from build123d import *

# Parameters (mm, degrees)
SKETCH1_W           = 35
SKETCH1_H           = 20
BOSS_EXTRUDE4_DEPTH = 15
SHELL2_T            = -2
SKETCH8_R           = 1.5
BOSS_EXTRUDE7_DEPTH = 6.9
LPATTERN4_COUNT     = 3
LPATTERN4_PITCH     = 10.5
FILLET1_R           = 2
CUT_EXTRUDE2_START  = -5
SKETCH9_R           = 1.25
CUT_EXTRUDE2_DEPTH  = 34.469380611
SKETCH10_R          = 1.25
CUT_EXTRUDE3_DEPTH  = 28.311380776


with BuildPart() as part:
    # Sketch1 → Boss-Extrude4 (new body)
    with BuildSketch(Plane(origin=(0, 0, 0), x_dir=(1, 0, 0), z_dir=(0, 1, 0))):
        Rectangle(SKETCH1_W, SKETCH1_H)
    extrude(amount=BOSS_EXTRUDE4_DEPTH)

    # Shell2
    shell2_openings = [part.faces().sort_by_distance(p)[0] for p in [
        (0, 15, 0),
    ]]
    offset(amount=SHELL2_T, openings=shell2_openings, kind=Kind.INTERSECTION)

    # Sketch8 → Boss-Extrude7 (add)
    with BuildSketch(Plane(origin=(13.95, 0, 0), x_dir=(0, 0, -1), z_dir=(1, 0, 0))):
        with BuildLine():
            Line((13.926543174, 13.400522246), (10, 9))
            Line((10, 9), (10, 15))
            ThreePointArc((10, 15), (13.096526294, 16.982277643), (13.926543174, 13.400522246))
        make_face()
        with Locations((12.249990037, 14.993304126)):
            Circle(SKETCH8_R, mode=Mode.SUBTRACT)
    boss_extrude7 = extrude(amount=-BOSS_EXTRUDE7_DEPTH)

    # LPattern4: Boss-Extrude7 ×3
    with Locations(*[(-i * LPATTERN4_PITCH, 0, 0) for i in range(1, LPATTERN4_COUNT)]):
        add(boss_extrude7)

    # Fillet1
    fillet1_edges = [part.edges().sort_by_distance(p)[0] for p in [
        (17.5, 7.5, 10),
        (-17.5, 7.5, 10),
    ]]
    fillet(fillet1_edges, radius=FILLET1_R)

    # Sketch9 → Cut-Extrude2 (cut)
    with BuildSketch(Plane(origin=(0, 0, 0), x_dir=(1, 0, 0), z_dir=(0, 1, 0)).offset(CUT_EXTRUDE2_START)):
        with Locations(Location((-4.997517741, 4.250548665, 0), (0, 0, 90))):
            Circle(SKETCH9_R)
    cut_extrude2 = extrude(amount=CUT_EXTRUDE2_DEPTH, mode=Mode.SUBTRACT)

    # Sketch10 → Cut-Extrude3 (cut, through all)
    with BuildSketch(Plane(origin=(0, 2, 0), x_dir=(1, 0, 0), z_dir=(0, 1, 0))):
        with Locations(Location((-5.055245898, -0.559104904, 0), (0, 0, 270))):
            Circle(SKETCH10_R)
    cut_extrude3 = extrude(amount=-CUT_EXTRUDE3_DEPTH, mode=Mode.SUBTRACT)

    # Mirror1: Cut-Extrude2, Cut-Extrude3 across plane
    add(cut_extrude2.mirror(Plane(origin=(0, 0, 0), x_dir=(0, 0, 1), z_dir=(1, 0, 0))), mode=Mode.SUBTRACT)
    add(cut_extrude3.mirror(Plane(origin=(0, 0, 0), x_dir=(0, 0, 1), z_dir=(1, 0, 0))), mode=Mode.SUBTRACT)


solid = part.part
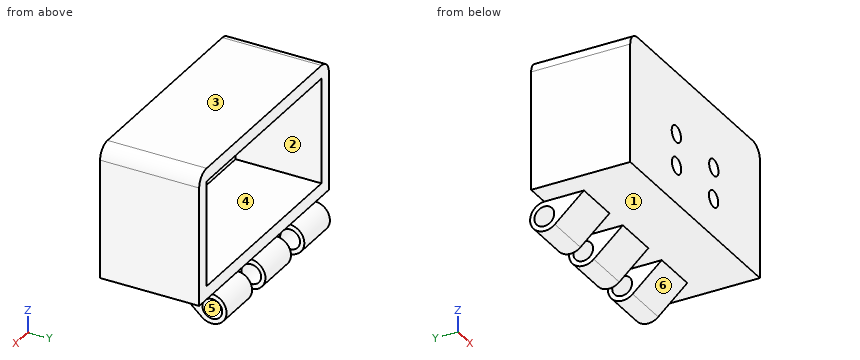
Design review of the part built by this model. Coordinates are the model's own, in mm. Face numbers are marked on the shaded views. A direction names the side the tool comes from. Round coordinates to 2 decimals unless told otherwise and drop trailing zeros. Write each loop counter-clockwise with the first axis right and the second up, starting at its lowest first coordinate (ties: lowest second). Pieces come first, ordered by that corner, then holes. Notation, with made-up numbers: (-22, 48) - (14, 48) arc R32 ccw to (14, 80) - close; hole circle Ø10 at (-5.5, 30). An arc over 180 degrees is marked (long way). Use a Markdown table: item, result. Add a question column.
1. We need section C-C (z = -4.5). State the section outline as (x, y) points, then the cut area to 3 significant figures.
2. Mouldability with a two-part tool opening along Y and no side actions: class the marked faces 4, 5 and 6 as +Y half, -Y half, draft (parallel to the pull), parting line (faces both ways), or undercut.
3. We need section B-B (z = -11.75). State the section outline as (x, y) points, then the cut area to 3 significant figures.
4. We need section D-D (x = 14.5). State the section outline as (y, z) points.
5. For the marked faces 1, 2 and 3, list the 3-axis set-ups (+Z, -Z, +X, -X, +Y, -Y) from which the entire face can be reached by the end or side of a thin tool; tool diameter is ignored.
6. Wall thickness on probe 1 along X at (y, z) = (9.25, 1.5); probe 2 along Z at (x, y) = (-15, 11.5); probe 3 along Z at (x, y) = (-10.5, 14): over which ranges is each line inside the solid? List them lowest first.
7. Clearance check with flat-ended pins moving along their axes: pin 1 (12 mm diameter, centred on x = -7.5, z = -4.5, fed in from +Y); pin 2 (2 mm diameter, centred on y = 13.5, z = -11.5, fed in from -X); pin 3 (1 mm diameter, centred on x = 2.5, y = 7.5, fed in from -Z); pin 4 (3 mm diameter, centred on x = -5.06, z = 0.56, fed in from -Y). State where each tip first meets the part, or that it passes through.
8. We need section A-A (y = 6.25). State the section outline as (x, z) points.
Output:
| question | item | result |
|---|---|---|
| 1 | outline | (-17.5, 0) - (-6.22, 0) - (-6.22, 2) - (-15.5, 2) - (-15.5, 15) - (-17.5, 15) - close; (-3.77, 0) - (3.77, 0) - (3.77, 2) - (-3.77, 2) - close; (6.22, 0) - (17.5, 0) - (17.5, 15) - (15.5, 15) - (15.5, 2) - (6.22, 2) - close |
| 1 | area | 112 mm2 |
| 2 | face 4 | draft |
| 2 | face 5 | undercut |
| 2 | face 6 | -Y half |
| 3 | outline | (-13.95, 10.96) - (-7.05, 10.96) - (-7.05, 13.58) - (-13.95, 13.58) - close; (-13.95, 16.41) - (-7.05, 16.41) - (-7.05, 17.09) - (-13.95, 17.09) - close; (-3.45, 10.96) - (3.45, 10.96) - (3.45, 13.58) - (-3.45, 13.58) - close; (-3.45, 16.41) - (3.45, 16.41) - (3.45, 17.09) - (-3.45, 17.09) - close; (7.05, 10.96) - (13.95, 10.96) - (13.95, 13.58) - (7.05, 13.58) - close; (7.05, 16.41) - (13.95, 16.41) - (13.95, 17.09) - (7.05, 17.09) - close |
| 3 | area | 68.4 mm2 |
| 4 | outline | (0, -10) - (15, -10) - (15, -8) - (2, -8) - (2, 8) - (15, 8) - (15, 10) - (0, 10) - close |
| 5 | face 1 | -Z, -Y |
| 5 | face 2 | +Y |
| 5 | face 3 | +Z, +X, -X, +Y, -Y |
| 6 | probe 1 | x = -17.5 to -15.5, 15.5 to 17.5 |
| 6 | probe 2 | z = -10 to -8, 8 to 10 |
| 6 | probe 3 | z = -14.31 to -13.37, -11.13 to -8, 8 to 10 |
| 7 | pin 1 | stops at y = 16.32 |
| 7 | pin 2 | stops at x = -13.95 |
| 7 | pin 3 | stops at z = -10 |
| 7 | pin 4 | stops at y = 0 |
| 8 | outline | (-17.5, -10) - (17.5, -10) - (17.5, 8) arc R2 ccw to (15.5, 10) - (-15.5, 10) arc R2 ccw to (-17.5, 8) - close; hole (-15.5, -8) - (15.5, -8) - (15.5, 8) - (-15.5, 8) - close |
